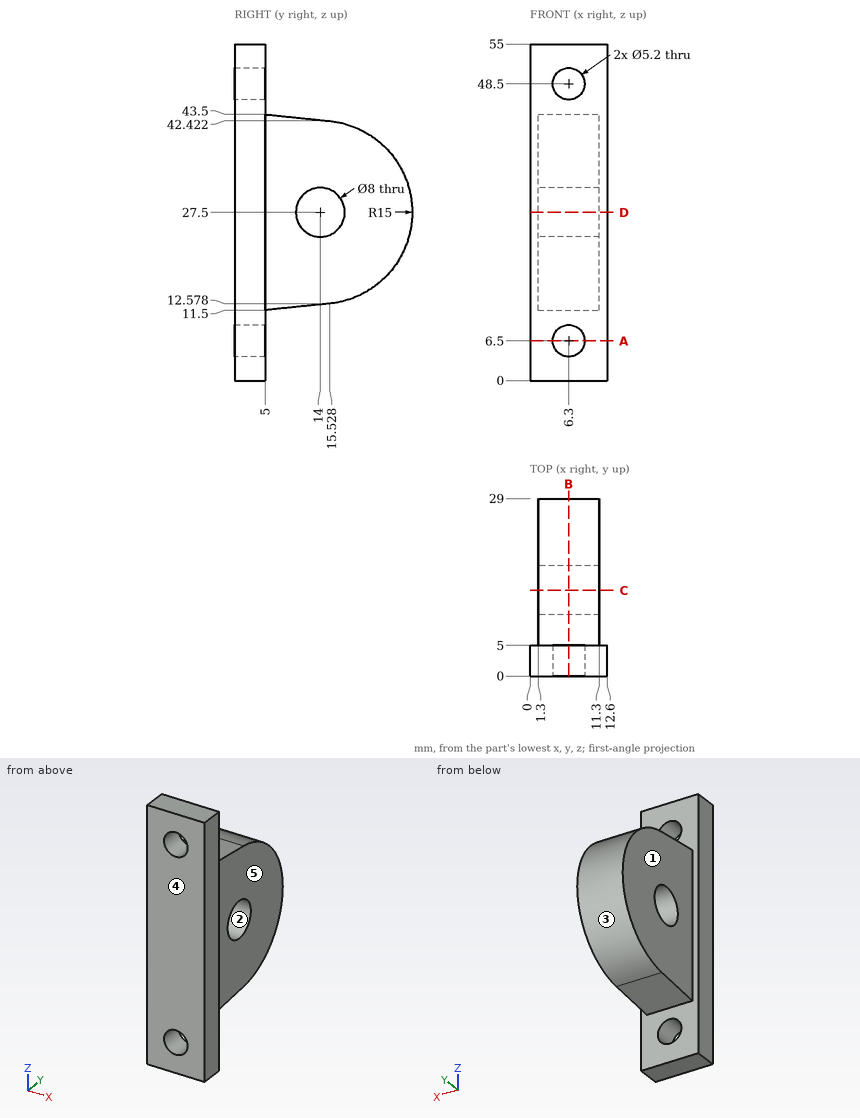
Geometry check sheet. Reference: drawing and pictorial views, mm from the part's lowest x, y, z. A direction names the side the tool comes from. Coordinates: 2 decimals unless noted, no trailing zeros. Order: outer loops, then holes, each group sorted by start corner. A loop starts at its lowest first (then second) coordinate and runs counter-clockwise, first axis right, second up. Notation, with made-up numbers: (29.25, 35.25) -> (62.25, 35.25) arc R23 cw to (62.25, 67.25) -> close; hole circle Ø7 at (-23.75, 77). An arc over 180 degrees is marked (long way). Use CSV: the item, a comma, the result in double quotes. Start each with the question number.
Q1. Thickness scan on line 1 along X through (y, z) = (3.4, 48.5); line 2 along Y through (x, z) = (8.5, 3.5); line 3 along X through (y, z) = (2.25, 5.5). Record the ranges inside material, lowest first.
Q2. Section check C-C, the plane y = 14. Record the cut outline in (x, z).
Q3. Section check B-B, the plane x = 6.3. Record the cut outline in (y, z).
Q4. Section check D-D, the plane z = 27.5. Record the cut outline in (x, y).
Q5. Tool access check on the marked faces 4 and 5. Record the directions out of +Z, -Z, +X, -X, +Y, -Y that give a thin tool (end or side, any length) a straight path to the whole face; none if there is none.
Q6. Section check A-A, the plane z = 6.5. Record the cut outline in (x, y).
Q7. Draft check along Z on the marked faces 1, 2 and 3. Enter one of: +Z half, -Z half, draft (parallel to the pull), parting line (faces both ways), or undercut.
Q8. Depth check by flat-ended pin: P1, Ø2, axis at x = 3, y = 9.5, coming from the +Z side; P2, Ø5, axis at x = 6, y = 15, coming from the -Z side; P3, Ø4.5, axis at x = 6.3, z = 48.5, coming from the -Y side; P4, Ø7, axis at y = 13.5, z = 27, coming from the -X side. Enter the tip coordinate at first touch or a pass-through.
Returned:
1,line 1,"x = 0 to 3.7, 8.9 to 12.6"
1,line 2,"y = 0 to 5"
1,line 3,"x = 0 to 3.9, 8.7 to 12.6"
2,outline,"(1.3, 12.42) -> (11.3, 12.42) -> (11.3, 23.5) -> (1.3, 23.5) -> close; (1.3, 31.5) -> (11.3, 31.5) -> (11.3, 42.58) -> (1.3, 42.58) -> close"
3,outline,"(0, 0) -> (5, 0) -> (5, 3.9) -> (0, 3.9) -> close; (0, 9.1) -> (5, 9.1) -> (5, 11.5) -> (15.53, 12.58) arc R15 ccw to (15.53, 42.42) -> (5, 43.5) -> (5, 45.9) -> (0, 45.9) -> close; (0, 51.1) -> (5, 51.1) -> (5, 55) -> (0, 55) -> close; hole circle Ø8 at (14, 27.5)"
4,outline,"(0, 0) -> (12.6, 0) -> (12.6, 5) -> (11.3, 5) -> (11.3, 10) -> (1.3, 10) -> (1.3, 5) -> (0, 5) -> close; (1.3, 18) -> (11.3, 18) -> (11.3, 29) -> (1.3, 29) -> close"
5,face 4,"+Z, -Z, +X, -X, -Y"
5,face 5,"+Z, -Z, +X, +Y"
6,outline,"(0, 0) -> (3.7, 0) -> (3.7, 5) -> (0, 5) -> close; (8.9, 0) -> (12.6, 0) -> (12.6, 5) -> (8.9, 5) -> close"
7,face 1,"draft"
7,face 2,"undercut"
7,face 3,"parting line"
8,P1,"stops at z = 43.14"
8,P2,"stops at z = 12.27"
8,P3,"passes through"
8,P4,"stops at x = 1.3"
